Job drawing, mm, ordinate dimensions from the low corner. One solid piece. A direction names the side the tool comes from. Coordinates: 2 decimals unless noted, no trailing zeros. Loops run counter-clockwise (first coordinate to the right, second up) from the corner with the lowest first, then second, coordinate; pieces in that order, holes last. Notation, with made-up numbers: M -19,20 L -12,20 A16 cw -12,48 Z; hole C 17,89.25 d7. An arc over 180 degrees is marked long. Answer as a JSON object with one key per item and string values. Group by question number.
1. Saw through at A-A on x = 73. Write the cut outline in (y, z), then the cut area to 3 significant figures.
2. Mould opens along Y. For the marked faces 4, 5 and 6 say: released by +Y, released by -Y, zero draft, split by the parting line, or undercut.
3. Drill centre lines: L1, parallel to Y at x = 93, z = 33; L2, parallel to Z at x = 77, y = 29; L3, parallel to X at y = 12.5, z = 7.5. Where is each one in solid material? Low to high.
4. Drop flat-ended pins along their axis: pin 1 Ø4 at (x, y) = (68, 40) entering from +Z; pin 2 Ø2 at (x, z) = (20, 9.5) entering from -Y; pin 3 Ø4.5 at (y, z) = (21.5, 6) entering from +X; pin 4 Ø12 at (y, z) = (10.5, 19) entering from -X. Give the stop position or say it passes through.
5. Saw through at C-C on y = 20. Write the cut outline in (x, z).
6. Saw through at D-D on z = 2. Write the cut outline in (x, y), then the cut area to 3 significant figures.
7. Saw through at B-B on z = 28.5. Write the cut outline in (x, y).
8. 3-axis set-ups, long thin cutter, end or side, ignore diameter. For the marked faces 1, 2 and 3: which of +Z, -Z, +X, -X, +Y, -Y reach the whole face in a straight line?
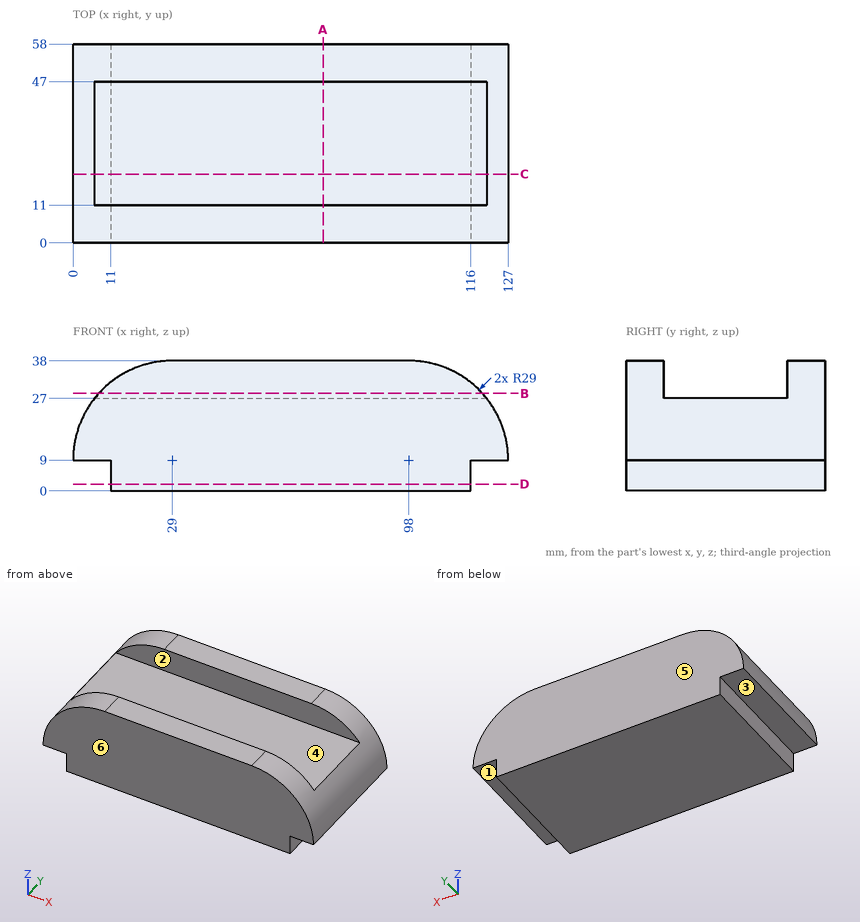
Outcome:
{
 "1": {"outline": "M 0,0 L 58,0 L 58,38 L 47,38 L 47,27 L 11,27 L 11,38 L 0,38 Z", "area": "1,810 mm²"},
 "2": {"face 4": "undercut", "face 5": "released by +Y", "face 6": "released by -Y"},
 "3": {"L1": "y = 0 to 11, 47 to 58", "L2": "z = 0 to 27", "L3": "x = 11 to 116"},
 "4": {"pin 1": "stops at z = 27", "pin 2": "stops at y = 0", "pin 3": "stops at x = 116", "pin 4": "stops at x = 0.28"},
 "5": {"outline": "M 0,9 L 11,9 L 11,0 L 116,0 L 116,9 L 127,9 A29 ccw 120.74,27 L 6.26,27 A29 ccw Z"},
 "6": {"outline": "M 11,0 L 116,0 L 116,58 L 11,58 Z", "area": "6,090 mm²"},
 "7": {"outline": "M 7.53,0 L 119.47,0 L 119.47,11 L 7.53,11 Z; M 7.53,47 L 119.47,47 L 119.47,58 L 7.53,58 Z"},
 "8": {"face 1": "-Z, +X, +Y, -Y", "face 2": "+Z, +X, -X", "face 3": "-Z, -X, +Y, -Y"}
}
